Can you work these out from the model? Positions are in its coordinate system, mm. A direction names the side the tool comes from. Coordinates: 2 decimals unless noted, no trailing zeros. Loops run counter-clockwise (first coordinate to the right, second up) from the corner with the lowest first, then second, coordinate; pieces in that order, holes last.
```python
from build123d import *

# Parameters (mm, degrees)
SKETCH021_R                          = 1.75
EXTRUDE005_DEPTH                     = 15
SKETCH020_W                          = 40
SKETCH020_H                          = 16
EXTRUDE003_DEPTH                     = 3
SKETCH016_AS_DRAWN_R                 = 13.5
EXTRUDE001_DEPTH                     = 45
EXTRUDE001_ONTO_SKETCH016_ROLL_ANGLE = 90
SKETCH017_AS_DRAWN_W                 = 6
SKETCH017_AS_DRAWN_H                 = 25
EXTRUDE002_DEPTH                     = 30
EXTRUDE002_ONTO_SKETCH017_ROLL_ANGLE = 90
EXTRUDE006_DEPTH                     = 15
EXTRUDE004_DEPTH                     = 3
SKETCH_R                             = 1.75
EXTRUDE_DEPTH                        = 38
SKETCH014_W                          = 22
SKETCH014_H                          = 20
BOX_W                                = 36
BOX_H                                = 60
BOX_DEPTH                            = 70


with BuildPart() as extrude005:
    # Sketch021 → Extrude005 (new body)
    with BuildSketch(Plane.XY):
        with Locations((-13.5, 56)):
            Circle(SKETCH021_R)
        with Locations((13.5, 56)):
            Circle(SKETCH021_R)
        with Locations((0, 50)):
            Circle(SKETCH021_R)
    extrude(amount=EXTRUDE005_DEPTH)


with BuildPart() as extrude005_1:
    # Extrude005 placement: moved
    add(extrude005.part.moved(Location((0, 0, 13))))


with BuildPart() as extrude003:
    # Sketch020 → Extrude003 (new body)
    with BuildSketch(Plane.XY):
        with Locations((0, 53)):
            Rectangle(SKETCH020_W, SKETCH020_H)
    extrude(amount=EXTRUDE003_DEPTH)


with BuildPart() as extrude003_1:
    # Extrude003 placement: moved
    add(extrude003.part.moved(Location((0, 0, 68))))


with BuildPart() as extrude_tube_hole:
    # Sketch016 as drawn → Extrude001 (new)
    with BuildSketch(Plane.XY):
        with Locations((0, 50)):
            Circle(SKETCH016_AS_DRAWN_R)
    extrude(amount=-EXTRUDE001_DEPTH)


with BuildPart() as extrude_tube_hole_1:
    # Extrude001 onto Sketch016 roll: moved
    add(extrude_tube_hole.part.rotate(Axis((0, 0, 0), (1, 0, 0)), EXTRUDE001_ONTO_SKETCH016_ROLL_ANGLE))


with BuildPart() as extrude_tube_hole_2:
    # Extrude001 onto Sketch016 placement: moved
    add(extrude_tube_hole_1.part)


with BuildPart() as extrude_tube_hole_3:
    # Extrude001 placement: moved
    add(extrude_tube_hole_2.part.moved(Location((0, -1, 0))))


with BuildPart() as arc_ext:
    # Sketch017 as drawn → Extrude002 (new)
    with BuildSketch(Plane.XY):
        with BuildLine():
            Line((8, 34), (20, 34))
            Line((20, 34), (20, 20))
            Line((20, 20), (7, 20))
            Line((7, 20), (7, 33))
            ThreePointArc((8, 34), (7.292893, 33.707107), (7, 33))
        make_face()
        with BuildLine():
            Line((-8, 34), (-20, 34))
            Line((-20, 34), (-20, 20))
            Line((-20, 20), (-7, 20))
            Line((-7, 20), (-7, 33))
            ThreePointArc((-7, 33), (-7.292893, 33.707107), (-8, 34))
        make_face()
        with Locations((0, 27.5)):
            Rectangle(SKETCH017_AS_DRAWN_W, SKETCH017_AS_DRAWN_H)
    extrude(amount=-EXTRUDE002_DEPTH)


with BuildPart() as arc_ext_1:
    # Extrude002 onto Sketch017 roll: moved
    add(arc_ext.part.rotate(Axis((0, 0, 0), (1, 0, 0)), EXTRUDE002_ONTO_SKETCH017_ROLL_ANGLE))


with BuildPart() as arc_ext_2:
    # Extrude002 onto Sketch017 placement: moved
    add(arc_ext_1.part)


with BuildPart() as arc_ext_3:
    # Extrude002 placement: moved
    add(arc_ext_2.part.moved(Location((0, -1, 0))))


with BuildPart() as extrude006:
    # Sketch021 → Extrude006 (new body)
    with BuildSketch(Plane.XY):
        with Locations((-13.5, 56)):
            Circle(SKETCH021_R)
        with Locations((13.5, 56)):
            Circle(SKETCH021_R)
        with Locations((0, 50)):
            Circle(SKETCH021_R)
    extrude(amount=EXTRUDE006_DEPTH)


with BuildPart() as extrude006_1:
    # Extrude006 placement: moved
    add(extrude006.part.moved(Location((0, 0, 58))))


with BuildPart() as extrude004:
    # Sketch020 → Extrude004 (new body)
    with BuildSketch(Plane.XY):
        with Locations((0, 53)):
            Rectangle(SKETCH020_W, SKETCH020_H)
    extrude(amount=EXTRUDE004_DEPTH)


with BuildPart() as extrude004_1:
    # Extrude004 placement: moved
    add(extrude004.part.moved(Location((0, 0, 14))))


with BuildPart() as fusion001:
    # Sketch → Extrude (new body)
    with BuildSketch(Plane.YZ):
        with Locations((10, 27.5)):
            Circle(SKETCH_R)
        with BuildLine():
            Line((61, 60), (47.5, 60))
            ThreePointArc((47.5, 60), (42.196699, 57.803301), (40, 52.5))
            Line((40, 52.5), (40, 32.5))
            ThreePointArc((40, 32.5), (42.196699, 27.196699), (47.5, 25))
            Line((47.5, 25), (61, 25))
            Line((61, 25), (61, 60))
        make_face()
        with BuildLine():
            Line((61, 15), (47.5, 15))
            ThreePointArc((47.5, 15), (42.196699, 12.803301), (40, 7.5))
            Line((40, 7.5), (40, -2))
            Line((40, -2), (61, -2))
            Line((61, -2), (61, 15))
        make_face()
        with BuildLine():
            Line((30, 50), (30, -2))
            Line((30, -2), (-2, -2))
            Line((-2, -2), (-2, 22))
            Line((-2, 22), (21, 22))
            Line((21, 22), (21, 50))
            ThreePointArc((30, 50), (25.5, 54.5), (21, 50))
        make_face()
    extrude(amount=EXTRUDE_DEPTH)


with BuildPart() as fusion001_1:
    # Extrude placement: moved
    add(fusion001.part.moved(Location((-19, 0, 0))))

    # Fusion001: union Extrude005, Extrude003, Extrude-tube-hole, arc-ext, Extrude006, Extrude004
    add(extrude005_1.part)
    add(extrude003_1.part)
    add(extrude_tube_hole_3.part)
    add(arc_ext_3.part)
    add(extrude006_1.part)
    add(extrude004_1.part)


with BuildPart() as sweep_body:
    # Sweep: sweep along a path in Sketch015
    with BuildLine(Plane.XZ) as sweep_path:
        ThreePointArc((4, 40.834849), (0, 60), (-4, 40.834849))
    # Sketch014 → Sweep (sweep)
    with BuildSketch(Plane(origin=(0, -1, 0), x_dir=(0, 1, 0), z_dir=(1, 0, 0))):
        with Locations((11, 78)):
            Rectangle(SKETCH014_W, SKETCH014_H)
    sweep(path=sweep_path.line)


with BuildPart() as fusion:
    # Sweep001: sweep along a path in Sketch019
    with BuildLine(Plane.XZ) as sweep001_path:
        ThreePointArc((10, 50), (0, 60), (-10, 50))
    # Sketch018 → Sweep001 (sweep)
    with BuildSketch(Plane(origin=(0, -1, 0), x_dir=(0, 1, 0), z_dir=(1, 0, 0))):
        Polygon((22, 68), (0, 68), (82.621778, 103), align=None)
    sweep(path=sweep001_path.line)

    # Fusion: union Sweep body
    add(sweep_body.part)


with BuildPart() as cut001:
    # Box → Box (new body)
    with BuildSketch(Plane(origin=(-18, 0, 0), x_dir=(1, 0, 0), z_dir=(0, 0, 1))):
        with Locations((18, 30)):
            Rectangle(BOX_W, BOX_H)
    extrude(amount=BOX_DEPTH)

    # Cut: cut Fusion
    add(fusion.part, mode=Mode.SUBTRACT)

    # Cut001: cut Fusion001
    add(fusion001_1.part, mode=Mode.SUBTRACT)


solid = cut001.part
```
(1) I'm going to push flat-ended pins straight in: pin 1 (8 mm diameter, centred on x = -11.5, z = 49.5, fed in from +Y); pin 2 (5.5 mm diameter, centred on y = 14.5, z = 30, fed in from -X); pin 3 (4 mm diameter, centred on x = -3, y = 54, fed in from +Z). Where does each tip first touch, or does it pass through?
Check values:
pin 1: stops at y = 40.03
pin 2: stops at x = -7
pin 3: stops at z = 68
(2) I want a section at A-A on x = 0. State how many separate pieces and enclosed holes the cut face has, then the cut area to 3 significant figures.
Check values:
separate pieces: 4
enclosed holes: 0
area: 874 mm2
(3) If I drill on probe 1 along X at (y, z) = (56, 23); probe 2 along Y at (x, z) = (-15, 48); probe 3 along Z at (x, y) = (-15, 49.5), over which ranges is the centre line in solid material (lowest first)?
Check values:
probe 1: x = -18 to -15.25, -11.75 to 11.75, 15.25 to 18
probe 2: y = 0 to 21, 30 to 40
probe 3: z = 17 to 25, 60 to 68
(4) I want a section at B-B on y = 10. Write out the boundary of the cut face in (x, z).
Check values:
outline: (-8.25, 34) - (-8, 34) arc R1 cw to (-7, 33) - (-7, 29.25) - (-3, 29.25) - (-3, 36.84) arc R13.5 cw (long way) to (3, 36.84) - (3, 29.25) - (7, 29.25) - (7, 33) arc R1 cw to (8, 34) - (8.25, 34) arc R18 ccw (long way) to start; (-7, 22) - (-3, 22) - (-3, 25.75) - (-7, 25.75) - close; (3, 22) - (7, 22) - (7, 25.75) - (3, 25.75) - close
(5) I want a section at D-D on z = 20. Write out the boundary of the cut face in (x, y), then the cut area to 3 significant figures.
Check values:
outline: (-18, 30) - (18, 30) - (18, 60) - (-18, 60) - close; hole circle Ø3.5 at (-13.5, 56); hole circle Ø3.5 at (0, 50); hole circle Ø3.5 at (13.5, 56)
area: 1,050 mm2
(6) I want a section at C-C on y = 50. Write out the boundary of the cut face in (x, z).
Check values:
outline: (-18, 17) - (-1.75, 17) - (-1.75, 25) - (-18, 25) - close; (-18, 60) - (-1.75, 60) - (-1.75, 68) - (-18, 68) - close; (1.75, 17) - (18, 17) - (18, 25) - (1.75, 25) - close; (1.75, 60) - (18, 60) - (18, 68) - (1.75, 68) - close
(7) Which directions (+Z, -Z, +X, -X, +Y, -Y) give clear straight access to the entire face, cutting with the end or side of a thin tool? Please do faces 5 (the flat face through (0, 53, 17)), 6 (the cylindrical face through (-0.252, 42.139, 27.255)), 7 (the flat face through (-3, 10, 31)).
Check values:
face 5: -Z, +X, -X, +Y
face 6: +X, -X, +Y
face 7: -Z, -Y
(8) If we mould it in two halves opening along Z, with no side actions, what happens to faces 1 (the flat face through (9, 21, 36)), 2 (the flat face through (0, 37, 70)), 3 (the flat face through (0, 35, 0)), 4 (the cylindrical face through (-0.252, 44.405, 59.332))? For each: released by +Z, released by -Z, zero draft, split by the parting line, or undercut.
Check values:
face 1: zero draft
face 2: released by +Z
face 3: released by -Z
face 4: undercut
